Geometry check sheet. Reference: the model listing, model coordinates, mm. A direction names the side the tool comes from. Round coordinates to 2 decimals unless told otherwise and drop trailing zeros. Loops run counter-clockwise (first coordinate to the right, second up) from the corner with the lowest first, then second, coordinate; pieces in that order, holes last. Notation, with made-up numbers: (-19.75, -33.75) -> (-7.75, -33.75) arc R26 ccw to (-7.75, 5.25) -> close; hole circle Ø11 at (-31, -12.5). An arc over 180 degrees is marked (long way). Use a Markdown table: item, result. Add a question column.
Q1. Release check for a two-part mould opening along X. For faces 1 (the face through (39, 11, 39)), 2 (the face through (44, 0, 41)), 3 (the face through (-58.398, 9.972, -12.968)) record: released by +X, released by -X, zero draft, split by the parting line, or undercut.
Q2. Material ranges on L1, parallel to X at y = 11.55, z = 0; L2, parallel to X at y = 3.75, z = 0; L3, parallel to Z at x = 49, y = 6.5, recorded low to high.
Q3. Set-up check for faces 4 (the face through (44, 0, -42)), 5 (the face through (43, 6, -22)), 6 (the face through (10.178, 7.909, 51.103)), 7 (the face through (-59, 8, 13)): record each of +Z, -Z, +X, -X, +Y, -Y from which the full face is reachable in a straight line by a thin tool's end or side.
Q4. Sectioned sample at A-A, the plane x = -7.5. Enter the section's corners in (y, z).
Q5. Gauge pin test, flat ends, axial feed: P1, Ø1, axis at y = 5.5, z = 12, coming from the +X side; P2, Ø1, axis at y = 6, z = 8.5, coming from the -X side; P3, Ø1, axis at x = -31.5, y = 5.5, coming from the +Z side. Record the tip position at first contact, or that the pin passes through.
```python
from build123d import *

# Parameters (mm, degrees)
SKETCH3_R                = 61.468
SKETCH3_R_2              = 58.95025584
BOSS_EXTRUDE1_DEPTH      = 8
SKETCH7_R                = 59.82025584
SKETCH7_R_2              = 58.95025584
BOSS_EXTRUDE2_DEPTH      = 4
CUT_EXTRUDE1_DEPTH       = 88.753233832
FILLET1_R                = 2.54
CIRPATTERN1_COUNT        = 4
FILLET1_OF_CIRPATTERN1_R = 2.54
CUT_EXTRUDE4_DEPTH       = 88.753233984
CIRPATTERN3_COUNT        = 4


with BuildPart() as part:
    # Sketch3 → Boss-Extrude1 (new body)
    with BuildSketch(Plane(origin=(0, 0, 0), x_dir=(1, 0, 0), z_dir=(0, 1, 0))):
        with Locations(Location((0, 0, 0), (0, 0, 270))):
            Circle(SKETCH3_R)
        with Locations(Location((0, 0, 0), (0, 0, 270))):
            Circle(SKETCH3_R_2, mode=Mode.SUBTRACT)
    extrude(amount=BOSS_EXTRUDE1_DEPTH)

    # Sketch7 → Boss-Extrude2 (add)
    with BuildSketch(Plane(origin=(0, 8, 0), x_dir=(1, 0, 0), z_dir=(0, 1, 0))):
        with Locations(Location((0, 0, 0), (0, 0, 270))):
            Circle(SKETCH7_R)
        with Locations(Location((0, 0, 0), (0, 0, 270))):
            Circle(SKETCH7_R_2, mode=Mode.SUBTRACT)
    extrude(amount=BOSS_EXTRUDE2_DEPTH)

    # Sketch9 → Cut-Extrude1 (cut, through all)
    with BuildSketch(Plane.XY):
        with BuildLine():
            Line((0, 0), (3, 0))
            ThreePointArc((3, 0), (0, 3), (-3, 0))
            Line((-3, 0), (0, 0))
        make_face()
    cut_extrude1 = extrude(amount=CUT_EXTRUDE1_DEPTH, mode=Mode.SUBTRACT)

    # Fillet1
    fillet1_edges = [part.edges().sort_by_distance(p)[0] for p in [
        (3, 0, 60.134309167),
        (-3, 0, 60.134309167),
    ]]
    fillet(fillet1_edges, radius=FILLET1_R)

    # CirPattern1: Cut-Extrude1 ×4 about axis
    cirpattern1_axis = Axis((0, 8, 0), (0, 1, 0))
    for i in range(1, CIRPATTERN1_COUNT):
        add(cut_extrude1.rotate(cirpattern1_axis, i * 360 / CIRPATTERN1_COUNT), mode=Mode.SUBTRACT)

    # Fillet1 of CirPattern1
    fillet1_of_cirpattern1_edges = [part.edges().sort_by_distance(p)[0] for p in [
        (60.134309167, 0, -3),
        (60.134309167, 0, 3),
        (-3, 0, -60.134309167),
        (3, 0, -60.134309167),
        (-60.134309167, 0, 3),
        (-60.134309167, 0, -3),
    ]]
    fillet(fillet1_of_cirpattern1_edges, radius=FILLET1_OF_CIRPATTERN1_R)

    # Sketch10 → Revolve2 (revolve)
    with BuildSketch(Plane.XY, mode=Mode.PRIVATE) as revolve2_sk:
        with BuildLine():
            Line((-58.95025584, 6), (-47.51025584, 6))
            ThreePointArc((-47.51025584, 6), (-51.004325155, 8.83618486), (-54.95025584, 11))
            Line((-54.95025584, 11), (-58.95025584, 11))
            Line((-58.95025584, 11), (-58.95025584, 6))
        make_face()
    revolve(revolve2_sk.sketch.rotate(Axis((0, 0, 0), (0, 1, 0)), 270), axis=Axis((0, 0, 0), (0, 1, 0)))

    # Sketch13 → Cut-Extrude4 (cut, through all)
    with BuildSketch(Plane(origin=(0, 0, 0), x_dir=(1, 0, 0), z_dir=(0, 1, 0))):
        with BuildLine():
            ThreePointArc((-9.707144427, 42.796913747), (-4.982712156, 44.461503222), (0, 44.97501853))
            Line((0, 44.97501853), (0, 55.25649697))
            ThreePointArc((0, 55.25649697), (-5.209883661, 54.933301733), (-10.339877075, 53.968672014))
            Line((-10.339877075, 53.968672014), (-9.707144427, 42.796913747))
        make_face()
        with BuildLine():
            Line((0, 55.25649697), (0, 44.97501853))
            ThreePointArc((0, 44.97501853), (4.993665079, 44.301497693), (9.688751248, 42.472157075))
            Line((9.688751248, 42.472157075), (10.339877075, 53.968672014))
            ThreePointArc((10.339877075, 53.968672014), (5.209883661, 54.933301733), (0, 55.25649697))
        make_face()
    cut_extrude4 = extrude(amount=CUT_EXTRUDE4_DEPTH, mode=Mode.SUBTRACT)

    # CirPattern3: Cut-Extrude4 ×4 about axis
    cirpattern3_axis = Axis((0, 0, 0), (0, 1, 0))
    for i in range(1, CIRPATTERN3_COUNT):
        add(cut_extrude4.rotate(cirpattern3_axis, i * 360 / CIRPATTERN3_COUNT), mode=Mode.SUBTRACT)


solid = part.part
```
Values:
| question | item | result |
|---|---|---|
| 1 | face 1 | undercut |
| 1 | face 2 | zero draft |
| 1 | face 3 | split by the parting line |
| 2 | L1 | -59.82 to -58.95, 58.95 to 59.82 |
| 2 | L2 | -61.47 to -58.95, 58.95 to 61.47 |
| 2 | L3 | -37.11 to -10.06, 10.06 to 37.11 |
| 3 | face 4 | +Z, -Z, +X, -X, -Y |
| 3 | face 5 | -Y |
| 3 | face 6 | +Y, -Y |
| 3 | face 7 | +Y |
| 4 | outline | (0, -61.01) -> (8, -61.01) -> (8, -59.35) -> (12, -59.35) -> (12, -58.47) -> (11, -58.47) -> (11, -54.58) -> (6, -54.58) -> (6, -58.47) -> (0, -58.47) -> close; (0, 58.47) -> (6, 58.47) -> (6, 54.58) -> (11, 54.58) -> (11, 58.47) -> (12, 58.47) -> (12, 59.35) -> (8, 59.35) -> (8, 61.01) -> (0, 61.01) -> close |
| 5 | P1 | x = 60.38 |
| 5 | P2 | x = -60.95 |
| 5 | P3 | z = 53.08 |
